```python
from build123d import *

# Parameters (mm, degrees)
SKETCH1_W           = 90
SKETCH1_H           = 45
BOSS_EXTRUDE1_DEPTH = 50
SKETCH2_R           = 4.15
CUT_EXTRUDE1_DEPTH  = 28.296664924
SKETCH3_R           = 7.65
CUT_EXTRUDE2_DEPTH  = 106.386194542
SKETCH4_R           = 1.5
CUT_EXTRUDE3_DEPTH  = 10
CHAMFER1_SIZE       = 1
SKETCH5_R           = 1.5
CUT_EXTRUDE4_DEPTH  = 10
SKETCH6_W           = 40
SKETCH6_H           = 20
CUT_EXTRUDE5_DEPTH  = 20
SKETCH7_R           = 5
CUT_EXTRUDE6_DEPTH  = 29


with BuildPart() as part:
    # Sketch1 → Boss-Extrude1 (new body)
    with BuildSketch(Plane(origin=(0, 0, 0), x_dir=(1, 0, 0), z_dir=(0, 1, 0))):
        Rectangle(SKETCH1_W, SKETCH1_H)
    extrude(amount=BOSS_EXTRUDE1_DEPTH)

    # Sketch2 → Cut-Extrude1 (cut)
    with BuildSketch(Plane.XY.offset(22.5)):
        with Locations((-30, 37.5)):
            Circle(SKETCH2_R)
        with Locations(Location((30, 37.5, 0), (0, 0, 180))):
            Circle(SKETCH2_R)
    extrude(amount=-CUT_EXTRUDE1_DEPTH, mode=Mode.SUBTRACT)

    # Sketch3 → Cut-Extrude2 (cut, through all)
    with BuildSketch(Plane(origin=(45, 0, 0), x_dir=(0, 0, -1), z_dir=(1, 0, 0))):
        with Locations((0, 12.5)):
            Circle(SKETCH3_R)
    extrude(amount=-CUT_EXTRUDE2_DEPTH, mode=Mode.SUBTRACT)

    # Sketch4 → Cut-Extrude3 (cut)
    with BuildSketch(Plane(origin=(45, 0, 0), x_dir=(0, 0, -1), z_dir=(1, 0, 0))):
        with Locations((-8.485281374, 20.985281374)):
            Circle(SKETCH4_R)
        with Locations((8.485281374, 20.985281374)):
            Circle(SKETCH4_R)
        with Locations((8.485281374, 4.014718626)):
            Circle(SKETCH4_R)
        with Locations((-8.485281374, 4.014718626)):
            Circle(SKETCH4_R)
    cut_extrude3 = extrude(amount=-CUT_EXTRUDE3_DEPTH, mode=Mode.SUBTRACT)

    # Mirror1: Cut-Extrude3 across plane
    add(cut_extrude3.mirror(Plane(origin=(0, 0, 0), x_dir=(0, 0, 1), z_dir=(1, 0, 0))), mode=Mode.SUBTRACT)

    # Chamfer1
    chamfer1_edges = [part.edges().sort_by_distance(p)[0] for p in [
        (-45, 50, 0),
        (0, 50, 22.5),
        (45, 50, 0),
        (0, 0, 22.5),
        (-45, 0, 0),
        (0, 0, -22.5),
        (45, 0, 0),
        (45, 25, 22.5),
        (-45, 25, 22.5),
        (-45, 25, -22.5),
        (45, 25, -22.5),
        (0, 50, -22.5),
    ]]
    chamfer(chamfer1_edges, length=CHAMFER1_SIZE)

    # Sketch5 → Cut-Extrude4 (cut)
    with BuildSketch(Plane(origin=(0, 50, 0), x_dir=(1, 0, 0), z_dir=(0, 1, 0))):
        with Locations(Location((15, 0.53825434, 0), (0, 0, 270))):
            Circle(SKETCH5_R)
        with Locations(Location((15, 17.53825434, 0), (0, 0, 270))):
            Circle(SKETCH5_R)
        with Locations(Location((-15, 17.53825434, 0), (0, 0, 90))):
            Circle(SKETCH5_R)
        with Locations(Location((-15, 0.53825434, 0), (0, 0, 90))):
            Circle(SKETCH5_R)
    extrude(amount=-CUT_EXTRUDE4_DEPTH, mode=Mode.SUBTRACT)

    # Sketch6 → Cut-Extrude5 (cut)
    with BuildSketch(Plane.XY.offset(22.5)):
        with Locations((0, 37)):
            Rectangle(SKETCH6_W, SKETCH6_H)
    extrude(amount=-CUT_EXTRUDE5_DEPTH, mode=Mode.SUBTRACT)

    # Sketch7 → Cut-Extrude6 (cut)
    with BuildSketch(Plane(origin=(0, 50, 0), x_dir=(1, 0, 0), z_dir=(0, 1, 0))):
        with Locations(Location((0, -14.241832216, 0), (0, 0, 90))):
            Circle(SKETCH7_R)
    extrude(amount=-CUT_EXTRUDE6_DEPTH, mode=Mode.SUBTRACT)


solid = part.part
```
Design review of the part built by this model. Coordinates are the model's own, in mm. A direction names the side the tool comes from. Coordinates: 2 decimals unless noted, no trailing zeros. Loops run counter-clockwise (first coordinate to the right, second up) from the corner with the lowest first, then second, coordinate; pieces in that order, holes last. Notation, with made-up numbers: (65, 66) -> (117, 66) arc R18 ccw to (117, 98) -> close; hole circle Ø7 at (-2.5, 28). An arc over 180 degrees is marked (long way). Answer as a JSON object with one key per item and string values.
Q1. Take a section at D-D on x = -30. Give the boundary of the cut face in (y, z).
Answer block:
{"outline": "(0, -21.5) -> (1, -22.5) -> (49, -22.5) -> (50, -21.5) -> (50, 21.5) -> (49, 22.5) -> (41.65, 22.5) -> (41.65, -5.8) -> (33.35, -5.8) -> (33.35, 22.5) -> (1, 22.5) -> (0, 21.5) -> close; hole circle Ø15.3 at (12.5, 0)"}
Q2. To check wall thickness, follow L1, parallel to Y at x = -18, z = 18.5; L2, parallel to X at y = 28, z = 8; L3, parallel to Y at x = -25, z = 0.5. State the ranges of each line that lie inside material, in increasing order.
Answer block:
{"L1": "y = 0 to 27, 47 to 50", "L2": "x = -45 to -20, 20 to 45", "L3": "y = 0 to 4.87, 20.13 to 50"}
Q3. Take a section at C-C on y = 12.5. Give the boundary of the cut face in (x, z), plus the area to 3 significant figures.
Answer block:
{"outline": "(-45, -21.5) -> (-44, -22.5) -> (44, -22.5) -> (45, -21.5) -> (45, -7.65) -> (-45, -7.65) -> close; (-45, 7.65) -> (45, 7.65) -> (45, 21.5) -> (44, 22.5) -> (-44, 22.5) -> (-45, 21.5) -> close", "area": "2,670 mm^2"}
Q4. The part is to be moulded in two halves that separate along Z. For faces 1 (the flat face through (-20, 37, 13)), 2 (the flat face through (30, 37, -5.797)), 3 (the cylindrical face through (-40.07, 19.52, 8.81)), say which applies: +Z half, -Z half, draft (parallel to the pull), parting line (faces both ways), or undercut.
Answer block:
{"face 1": "draft", "face 2": "+Z half", "face 3": "undercut"}
Q5. Clearance check with flat-ended pins moving along their axes: pin 1 Ø1.5 at (y, z) = (9, 4) entering from +X; pin 2 Ø9 at (x, z) = (0, 14.24) entering from +Y; pin 3 Ø1.8 at (y, z) = (20.99, 8.49) entering from -X. State where each tip first meets the part, or that it passes through.
Answer block:
{"pin 1": "passes through", "pin 2": "stops at y = 21", "pin 3": "stops at x = -35"}
Q6. Take a section at B-B on y = 25.5. Give the boundary of the cut face in (x, z), plus the area to 3 significant figures.
Answer block:
{"outline": "(-45, -21.5) -> (-44, -22.5) -> (44, -22.5) -> (45, -21.5) -> (45, 21.5) -> (44, 22.5) -> (-44, 22.5) -> (-45, 21.5) -> close; hole circle Ø10 at (0, 14.24)", "area": "3,970 mm^2"}
Q7. Take a section at A-A on x = 0. Give the boundary of the cut face in (y, z).
Answer block:
{"outline": "(0, -21.5) -> (1, -22.5) -> (49, -22.5) -> (50, -21.5) -> (50, 9.24) -> (47, 9.24) -> (47, 2.5) -> (27, 2.5) -> (27, 9.24) -> (21, 9.24) -> (21, 19.24) -> (27, 19.24) -> (27, 22.5) -> (1, 22.5) -> (0, 21.5) -> close; (47, 19.24) -> (50, 19.24) -> (50, 21.5) -> (49, 22.5) -> (47, 22.5) -> close; hole circle Ø15.3 at (12.5, 0)"}
Q8. Tool access review of faces 4 (the cylindrical face through (-1.502, 24.042, 9.473)), 5 (the cylindrical face through (40.1, 5.5, 8.7)), 6 (the cylindrical face through (-40.07, 5.5, -8.29)), 7 (the cylindrical face through (-27.77, 41, 8.55)), 8 (the flat face through (45, 25, 0)): name each direction out of +Z, -Z, +X, -X, +Y, -Y from which nothing blocks a thin tool from reaching the whole face with its end or side.
Answer block:
{"face 4": "+Y", "face 5": "+X", "face 6": "-X", "face 7": "+Z", "face 8": "+Z, -Z, +X, +Y, -Y"}
